Verification items for the finished model (mm, model axes). A direction names the side the tool comes from. Give positions to 0.01 mm unless a question says otherwise; leave off trailing zeros. Write each loop counter-clockwise with the first axis right and the second up, starting at its lowest first coordinate (ties: lowest second). Pieces come first, ordered by that corner, then holes. Notation, with made-up numbers: (-19.5, 83.25) - (1.5, 83.25) arc R11 cw to (1.5, 91.25) - close; hole circle Ø1 at (81.25, 52.25). An arc over 180 degrees is marked (long way). Put each result on its own line as item: value.
from build123d import *

# Parameters (mm, degrees)
SKETCH1_W           = 143
SKETCH1_H           = 176
BOSS_EXTRUDE1_DEPTH = 60
FILLET1_R           = 3
FILLET2_R           = 3
SHELL1_T            = -1
SKETCH2_R           = 17.5
CUT_EXTRUDE1_DEPTH  = 60


with BuildPart() as part:
    # Sketch1 → Boss-Extrude1 (new body)
    with BuildSketch(Plane(origin=(0, 0, 0), x_dir=(1, 0, 0), z_dir=(0, 1, 0))):
        Rectangle(SKETCH1_W, SKETCH1_H)
    extrude(amount=BOSS_EXTRUDE1_DEPTH)

    # Fillet1
    fillet1_edges = [part.edges().sort_by_distance(p)[0] for p in [
        (71.5, 30, 88),
        (-71.5, 30, 88),
        (-71.5, 30, -88),
        (71.5, 30, -88),
    ]]
    fillet(fillet1_edges, radius=FILLET1_R)

    # Fillet2
    fillet2_edges = [part.edges().sort_by_distance(p)[0] for p in [
        (0, 0, 88),
        (71.5, 0, 0),
        (-71.5, 0, 0),
        (0, 0, -88),
        (-70.621320344, 0, -87.121320344),
        (70.621320344, 0, -87.121320344),
        (70.621320344, 0, 87.121320344),
        (-70.621320344, 0, 87.121320344),
    ]]
    fillet(fillet2_edges, radius=FILLET2_R)

    # Shell1
    shell1_openings = [part.faces().sort_by_distance(p)[0] for p in [
        (0, 60, 0),
    ]]
    offset(amount=SHELL1_T, openings=shell1_openings, kind=Kind.INTERSECTION)

    # Sketch2 → Cut-Extrude1 (cut)
    with BuildSketch(Plane(origin=(71.5, 0, 0), x_dir=(0, 0, -1), z_dir=(1, 0, 0))):
        with Locations((45, 31.5)):
            Circle(SKETCH2_R)
    extrude(amount=-CUT_EXTRUDE1_DEPTH, mode=Mode.SUBTRACT)


solid = part.part
Q1. Release check for a two-part mould opening along X. For faces 1 (the face through (-1, 31, -87)), 2 (the face through (-1, 1, -1)), 3 (the face through (-1, 31, -88)), 4 (the face through (71.5, 31, 1)) record: released by +X, released by -X, zero draft, split by the parting line, or undercut.
Answers follow:
face 1: undercut
face 2: undercut
face 3: zero draft
face 4: released by +X
Q2. Go/stop test with a flat-tipped pin: pin 1 Ø4 at (x, z) = (-14.5, -32.5) entering from +Y. Record where the tip stops, or that it passes through.
Answers follow:
pin 1: stops at y = 1
Q3. Section check D-D, the plane z = 19. Record the cut outline in (x, y), plus the area to 3 significant figures.
Answers follow:
outline: (-71.5, 3) arc R3 ccw to (-68.5, 0) - (68.5, 0) arc R3 ccw to (71.5, 3) - (71.5, 60) - (70.5, 60) - (70.5, 3) arc R2 cw to (68.5, 1) - (-68.5, 1) arc R2 cw to (-70.5, 3) - (-70.5, 60) - (-71.5, 60) - close
area: 259 mm2
Q4. Section check A-A, the plane z = -45. Record the cut outline in (x, y).
Answers follow:
outline: (-71.5, 3) arc R3 ccw to (-68.5, 0) - (68.5, 0) arc R3 ccw to (71.5, 3) - (71.5, 14) - (70.5, 14) - (70.5, 3) arc R2 cw to (68.5, 1) - (-68.5, 1) arc R2 cw to (-70.5, 3) - (-70.5, 60) - (-71.5, 60) - close; (70.5, 49) - (71.5, 49) - (71.5, 60) - (70.5, 60) - close
Q5. Section check B-B, the plane y = 31.5. Record the cut outline in (x, z), plus the area to 3 significant figures.
Answers follow:
outline: (-71.5, -85) arc R3 ccw to (-68.5, -88) - (68.5, -88) arc R3 ccw to (71.5, -85) - (71.5, -62.5) - (70.5, -62.5) - (70.5, -85) arc R2 cw to (68.5, -87) - (-68.5, -87) arc R2 cw to (-70.5, -85) - (-70.5, 85) arc R2 cw to (-68.5, 87) - (68.5, 87) arc R2 cw to (70.5, 85) - (70.5, -27.5) - (71.5, -27.5) - (71.5, 85) arc R3 ccw to (68.5, 88) - (-68.5, 88) arc R3 ccw to (-71.5, 85) - close
area: 595 mm2
Q6. Section check C-C, the plane x = 46.5. Record the cut outline in (y, z).
Answers follow:
outline: (0, -85) arc R3 ccw to (3, -88) - (60, -88) - (60, -87) - (3, -87) arc R2 cw to (1, -85) - (1, 85) arc R2 cw to (3, 87) - (60, 87) - (60, 88) - (3, 88) arc R3 ccw to (0, 85) - close
Q7. Scan lines: line 1 along Z through (x, y) = (-46, 40); line 2 along X through (y, z) = (33, 72.5); line 3 along Y through (x, z) = (57.5, 77). Record each from-to range of solid material in increasing order.
Answers follow:
line 1: z = -88 to -87, 87 to 88
line 2: x = -71.5 to -70.5, 70.5 to 71.5
line 3: y = 0 to 1
Q8. Set-up check for faces 5 (the face through (71.007, 46.256, -54.408)), 6 (the face through (-1, 31, 88)), 7 (the face through (70.5, 31, 1)): record each of +Z, -Z, +X, -X, +Y, -Y from which the full face is reachable in a straight line by a thin tool's end or side.
Answers follow:
face 5: +X
face 6: +Z, +X, -X, +Y, -Y
face 7: +Y
